Can you work these out from the model? Positions are in its coordinate system, mm. Round coordinates to 2 decimals unless told otherwise and drop trailing zeros. Loops run counter-clockwise (first coordinate to the right, second up) from the corner with the lowest first, then second, coordinate; pieces in that order, holes last. Notation, with made-up numbers: (64.25, -37.75) -> (117.25, -37.75) arc R21 cw to (117.25, -21.75) -> close; hole circle Ø4 at (50.5, 18.25). An arc over 180 degrees is marked (long way). Write each question's results on one line, items separated by ' | '.
from build123d import *

# Parameters (mm, degrees)
PAD_DEPTH     = 10
FILLET001_1_R = 1
FILLET001_2_R = 0.7
BOX_W         = 200
BOX_H         = 6
BOX_DEPTH     = 3
FILLET_R      = 1.2


with BuildPart() as end_fillet:
    # Sketch → Pad (new body)
    with BuildSketch(Plane.XZ):
        Polygon((0, 0), (0, 3), (10, 0.5), (10, 0), align=None)
    extrude(amount=PAD_DEPTH)


with BuildPart() as end_fillet_1:
    # Body placement: moved
    add(end_fillet.part.moved(Location((0, 8, 0))))

    # Fillet001 1
    fillet001_1_edges = [end_fillet_1.edges().sort_by_distance(p)[0] for p in [
        (0, -2, 1.5),
    ]]
    fillet(fillet001_1_edges, radius=FILLET001_1_R)

    # Fillet001 2
    fillet001_2_edges = [end_fillet_1.edges().sort_by_distance(p)[0] for p in [
        (0, 8, 1.5),
    ]]
    fillet(fillet001_2_edges, radius=FILLET001_2_R)


with BuildPart() as fusion:
    # Box → Box (new body)
    with BuildSketch(Plane(origin=(-200, 0, 0), x_dir=(1, 0, 0), z_dir=(0, 0, 1))):
        with Locations((100, 3)):
            Rectangle(BOX_W, BOX_H)
    extrude(amount=BOX_DEPTH)

    # Fillet
    fillet_edges = [fusion.edges().sort_by_distance(p)[0] for p in [
        (-200, 0, 1.5),
        (-200, 6, 1.5),
    ]]
    fillet(fillet_edges, radius=FILLET_R)

    # Fusion: union end fillet
    add(end_fillet_1.part)


solid = fusion.part
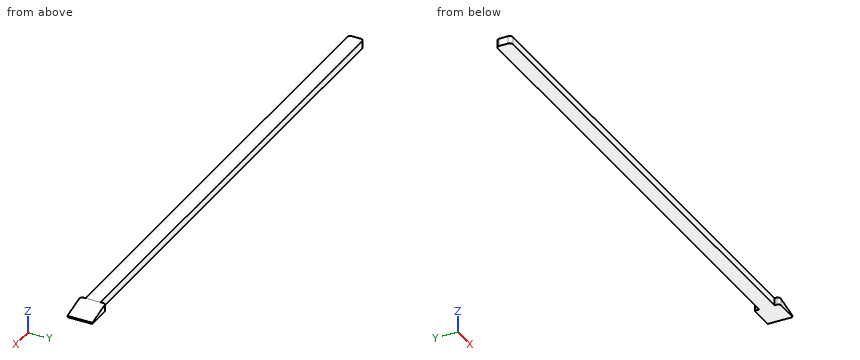
1. Please list where these lines run through material, in increasing order: line 1 (Y direction, x = -147.5, z = 2.4); line 2 (X direction, y = 6.75, z = 0.25); line 3 (X direction, y = 7.75, z = 0.2). Write a range as from..to.
Final values:
line 1: 0..6 | line 2: 0..10 | line 3: 0.16..10
2. Will these pins go through, and if not, where does the flat tip stop? pin 1 (1.4 mm diameter, centred on y = 7, z = 1, fed in from -X); pin 2 (1.5 mm diameter, centred on x = -115.5, z = 2, fed in from -Y); pin 3 (0.9 mm diameter, centred on x = -62.5, z = 1.5, fed in from +Y); pin 4 (1.5 mm diameter, centred on x = -71, y = -1, fed in from -Z).
Final values:
pin 1: x = 0 | pin 2: y = 0 | pin 3: y = 6 | pin 4: through
3. If we section it at B-B (x = -183): List the corners of the cut face in (y, z) for me, then the cut area to 3 significant figures.
Final values:
outline: (0, 0) -> (6, 0) -> (6, 3) -> (0, 3) -> close | area: 18.0 mm2
4. If we section it at A-A (z = 2): List the corners of the cut face in (x, y) for me, then the cut area to 3 significant figures.
Final values:
outline: (-200, 1.2) arc R1.2 ccw to (-198.8, 0) -> (0, 0) -> (0, -1) arc R1 ccw to (1, -2) -> (4, -2) -> (4, 8) -> (0.7, 8) arc R0.7 ccw to (0, 7.3) -> (0, 6) -> (-198.8, 6) arc R1.2 ccw to (-200, 4.8) -> close | area: 1,240 mm2
